```python
from build123d import *

# Parameters (mm, degrees)
BOSS_EXTRUDE1_DEPTH = 6.35
SKETCH4_W           = 88.9
SKETCH4_H           = 6.35
CUT_EXTRUDE2_DEPTH  = 401.905830589
FILLET2_R           = 25.4
SKETCH6_W           = 6.35
SKETCH6_H           = 152.4
CUT_EXTRUDE3_DEPTH  = 401.905830589
SKETCH7_W           = 6
SKETCH7_H           = 10
SKETCH7_R           = 1.8
CUT_EXTRUDE4_DEPTH  = 401.905830589


with BuildPart() as part:
    # Sketch1 → Boss-Extrude1 (new body)
    with BuildSketch(Plane(origin=(0, 0, 0), x_dir=(1, 0, 0), z_dir=(0, 1, 0))):
        with BuildLine():
            ThreePointArc((-304.8, -133.35), (-203.058992682, -158.608992682), (-177.8, -260.35))
            Line((-177.8, -260.35), (177.8, -260.35))
            ThreePointArc((177.8, -260.35), (203.058992682, -158.608992682), (304.8, -133.35))
            Line((304.8, -133.35), (304.8, 133.35))
            ThreePointArc((304.8, 133.35), (203.058992682, 158.608992682), (177.8, 260.35))
            Line((177.8, 260.35), (-177.8, 260.35))
            ThreePointArc((-177.8, 260.35), (-203.058992682, 158.608992682), (-304.8, 133.35))
            Line((-304.8, 133.35), (-304.8, -133.35))
        make_face()
    extrude(amount=BOSS_EXTRUDE1_DEPTH)

    # Sketch4 → Cut-Extrude2 (cut, through all)
    with BuildSketch(Plane(origin=(0, 6.35, 0), x_dir=(1, 0, 0), z_dir=(0, 1, 0))):
        with Locations((-177.8, 257.175)):
            Rectangle(SKETCH4_W, SKETCH4_H)
        with Locations((0, 257.175)):
            Rectangle(SKETCH4_W, SKETCH4_H)
        with Locations((177.8, 257.175)):
            Rectangle(SKETCH4_W, SKETCH4_H)
    cut_extrude2 = extrude(amount=-CUT_EXTRUDE2_DEPTH, mode=Mode.SUBTRACT)

    # Mirror2: Cut-Extrude2 across plane
    add(cut_extrude2.mirror(Plane.XY), mode=Mode.SUBTRACT)

    # Fillet2
    fillet2_edges = [part.edges().sort_by_distance(p)[0] for p in [
        (-304.8, 3.175, 133.35),
        (-304.8, 3.175, -133.35),
        (304.8, 3.175, -133.35),
        (304.8, 3.175, 133.35),
    ]]
    fillet(fillet2_edges, radius=FILLET2_R)

    # Sketch6 → Cut-Extrude3 (cut, through all)
    with BuildSketch(Plane(origin=(0, 6.35, 0), x_dir=(1, 0, 0), z_dir=(0, 1, 0))):
        with Locations((-200.025, 0)):
            Rectangle(SKETCH6_W, SKETCH6_H)
        with Locations((200.025, 0)):
            Rectangle(SKETCH6_W, SKETCH6_H)
    extrude(amount=-CUT_EXTRUDE3_DEPTH, mode=Mode.SUBTRACT)

    # Sketch7 → Cut-Extrude4 (cut, through all)
    with BuildSketch(Plane(origin=(0, 6.35, 0), x_dir=(1, 0, 0), z_dir=(0, 1, 0))):
        with Locations((11, 4)):
            Rectangle(SKETCH7_W, SKETCH7_H)
        with Locations(Location((-19.5, 25.5, 0), (0, 0, 270))):
            Circle(SKETCH7_R)
        with Locations(Location((-19.5, -25.5, 0), (0, 0, 90))):
            Circle(SKETCH7_R)
        with Locations(Location((19.5, -25.5, 0), (0, 0, 270))):
            Circle(SKETCH7_R)
        with Locations(Location((19.5, 25.5, 0), (0, 0, 90))):
            Circle(SKETCH7_R)
    extrude(amount=-CUT_EXTRUDE4_DEPTH, mode=Mode.SUBTRACT)


solid = part.part
```
The listing builds one solid part. Answer for the finished solid, in the listing's coordinates (mm). Coordinates: 2 decimals unless noted, no trailing zeros. Write each loop counter-clockwise with the first axis right and the second up, starting at its lowest first coordinate (ties: lowest second). Pieces come first, ordered by that corner, then holes. Notation, with made-up numbers: (67.25, 72) - (107.25, 72) arc R21 cw to (107.25, 85) - close; hole circle Ø9 at (12, 39). An arc over 180 degrees is marked (long way). Return JSON: item names as keys, results as strings. Group by question number.
Q1. The part is cut by section B-B on z = -211. Write down the section's boundary in (x, y).
Q2. For a pull along Z with two mould halves and no side action, classify faces 1 (the cylindrical face through (-296.833, 3.219, 122.004)), 2 (the cylindrical face through (296.833, 3.219, -122.004)), 3 (the flat face through (-4, 0, -4)), 4 (the cylindrical face through (195.47, 3.13, 167.1)) as +Z half, -Z half, draft (parallel to the pull), parting line (faces both ways), or undercut.
Q3. Flat-ended cylindrical pins translate along their axes: pin 1 Ø6 at (x, z) = (139, -11) entering from -Y; pin 2 Ø1.9 at (y, z) = (2.5, 258) entering from +X; pin 3 Ø1.5 at (x, y) = (184, 5.5) entering from +Z; pin 4 Ø2 at (x, z) = (-19.5, 25.5) entering from +Y. Find the tip coordinate at first contact, or state that the pin passes through.
Q4. Find the intervals of material crossed by line 1 along X through (y, z) = (2.75, -70); line 2 along X through (y, z) = (3, 25.5); line 3 along Z through (x, y) = (146.5, 4.5), in increasing order. Write a range as [from, to].
Q5. The part is cut by section A-A on y = 1.75. State how many separate pieces and enclosed holes the cut face has, and give its area (3 significant figures).
Q6. The part is cut by section C-C on x = 210.5. Write down the section's boundary in (y, z).
Evaluation:
{
 "1": {"outline": "(-175.18, 0) - (175.18, 0) - (175.18, 6.35) - (-175.18, 6.35) - close"},
 "2": {"face 1": "+Z half", "face 2": "-Z half", "face 3": "draft", "face 4": "undercut"},
 "3": {"pin 1": "stops at y = 0", "pin 2": "stops at x = 133.35", "pin 3": "stops at z = 186.6", "pin 4": "passes through"},
 "4": {"line 1": "x = [-304.8, -203.2], [-196.85, 196.85], [203.2, 304.8]", "line 2": "x = [-304.8, -203.2], [-196.85, -21.3], [-17.7, 17.7], [21.3, 196.85], [203.2, 304.8]", "line 3": "z = [-254, 254]"},
 "5": {"separate pieces": "1", "enclosed holes": "7", "area": "252,000 mm2"},
 "6": {"outline": "(0, -151.87) - (6.35, -151.87) - (6.35, 151.87) - (0, 151.87) - close"}
}
